The listing builds one solid part. Answer for the finished solid, in the listing's coordinates (mm). Face numbers are marked on the shaded views. A direction names the side the tool comes from. Round coordinates to 2 decimals unless told otherwise and drop trailing zeros. Write each loop counter-clockwise with the first axis right and the second up, starting at its lowest first coordinate (ties: lowest second). Pieces come first, ordered by that corner, then holes. Notation, with made-up numbers: (67, 20) - (110, 20) arc R19 cw to (110, 56) - close; hole circle Ø11 at (-21.75, 40). An arc over 180 degrees is marked (long way). Return JSON: item names as keys, results as strings. Group by question number.
(1) Section D-D, the plane z = -12 is taken. Write down the section's boundary in (x, y), then the cut area to 3 significant figures.
(2) Section A-A, the plane z = 0 is taken. Write down the section's boundary in (x, y).
(3) Find the intervals of material crossed by line 1 along Y through (x, z) = (7, 0); line 2 along X through (y, z) = (14.5, -14); line 3 along Y through (x, z) = (3, 0), in increasing order. Write a range as [from, to].
(4) Each of these flat-tipped pins is pushed along its axis until it touches: pin 1 (1.5 mm diameter, centred on x = 9, z = 0, fed in from +Y); pin 2 (1.5 mm diameter, centred on x = 29.5, y = 5.5, fed in from +Z); pin 3 (2 mm diameter, centred on y = 20, z = -20, fed in from +X); pin 4 (12 mm diameter, centred on x = 19, z = 16, fed in from -Y). Where does it stop, or does it pass through?
(5) Section C-C, the plane y = 0 is taken. Write down the section's boundary in (x, z), then the cut area to 3 significant figures.
(6) Section B-B, the plane y = 20 is taken. Write down the section's boundary in (x, z), then the cut area to 3 significant figures.
(7) Determine the mould class of the marked faces 1, 2 and 3 for opening direction X: +X half, -X half, draft (parallel to the pull), parting line (faces both ways), or undercut.
(8) Which of the six approach directions +Z, -Z, +X, -X, +Y, -Y give full straight-line access (tool end or side, diameter ignored) to the marked faces 4 and 5?
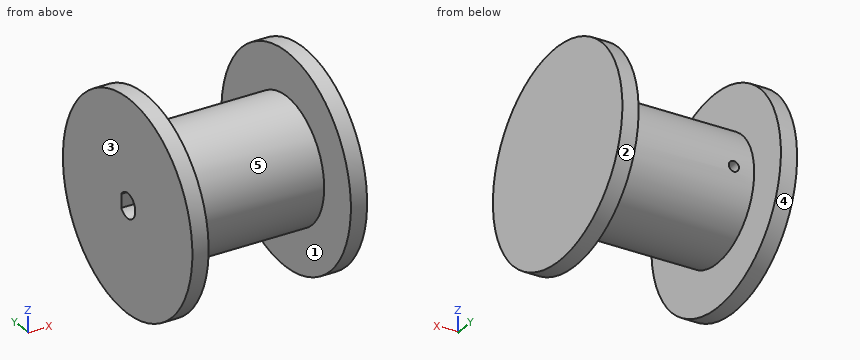
```python
from build123d import *

# Parameters (mm, degrees)
SKETCH7_W          = 1.25
SKETCH7_H          = 15
CUT_EXTRUDE1_DEPTH = 12


with BuildPart() as part:
    # Sketch1 → Revolve1 (revolve)
    with BuildSketch(Plane.XY, mode=Mode.PRIVATE) as revolve1_sk:
        Polygon((0, 0), (0, 3), (0, 25.5), (4, 25.5), (4, 15), (39, 15), (39, 25.5), (43, 25.5), (43, 3), (43, 0), align=None)
    revolve(revolve1_sk.sketch.rotate(Axis((0, 0, 0), (1, 0, 0)), 90), axis=Axis((0, 0, 0), (1, 0, 0)))

    # Sketch7 → M3 Tapped Hole1 (revolve, cut)
    with BuildSketch(Plane(origin=(9, 0, 0), x_dir=(0, 0, -1), z_dir=(1, 0, 0))):
        with Locations((0.625, 7.5)):
            Rectangle(SKETCH7_W, SKETCH7_H)
    revolve(axis=Axis((9, -6.35, 0), (0, 1, 0)), mode=Mode.SUBTRACT)

    # Sketch8 → Cut-Extrude1 (cut)
    with BuildSketch(Plane.ZY):
        with BuildLine():
            Line((-1.658312395, 2.5), (1.658312395, 2.5))
            ThreePointArc((1.658312395, 2.5), (0, -3), (-1.658312395, 2.5))
        make_face()
    extrude(amount=-CUT_EXTRUDE1_DEPTH, mode=Mode.SUBTRACT)


solid = part.part
```
Working result:
{
 "1": {"outline": "(0, -22.5) - (4, -22.5) - (4, -9) - (39, -9) - (39, -22.5) - (43, -22.5) - (43, 22.5) - (39, 22.5) - (39, 9) - (4, 9) - (4, 22.5) - (0, 22.5) - close", "area": "990 mm^2"},
 "2": {"outline": "(0, -25.5) - (4, -25.5) - (4, -15) - (39, -15) - (39, -25.5) - (43, -25.5) - (43, 25.5) - (39, 25.5) - (39, 15) - (10.25, 15) - (10.25, 2.5) - (12, 2.5) - (12, -3) - (0, -3) - close; (0, 2.5) - (7.75, 2.5) - (7.75, 15) - (4, 15) - (4, 25.5) - (0, 25.5) - close"},
 "3": {"line 1": "y = [-15, -3], [2.5, 15]", "line 2": "x = [0, 4], [39, 43]", "line 3": "y = [-25.5, -3], [2.5, 25.5]"},
 "4": {"pin 1": "stops at y = -2.9", "pin 2": "stops at z = 14.23", "pin 3": "passes through", "pin 4": "stops at y = -11.18"},
 "5": {"outline": "(0, -25.5) - (4, -25.5) - (4, -15) - (39, -15) - (39, -25.5) - (43, -25.5) - (43, 25.5) - (39, 25.5) - (39, 15) - (4, 15) - (4, 25.5) - (0, 25.5) - (0, 3) - (12, 3) - (12, -3) - (0, -3) - close", "area": "1,390 mm^2"},
 "6": {"outline": "(0, -15.82) - (4, -15.82) - (4, 15.82) - (0, 15.82) - close; (39, -15.82) - (43, -15.82) - (43, 15.82) - (39, 15.82) - close", "area": "253 mm^2"},
 "7": {"face 1": "undercut", "face 2": "draft", "face 3": "-X half"},
 "8": {"face 4": "+X, -X", "face 5": "none"}
}
